Geometry: final body of the model. Coordinates: model frame, mm. A direction names the side the tool comes from. Coordinates: 2 decimals unless noted, no trailing zeros. Write each loop counter-clockwise with the first axis right and the second up, starting at its lowest first coordinate (ties: lowest second). Pieces come first, ordered by that corner, then holes. Notation, with made-up numbers: (-10, 21) -> (-3, 21) arc R12 cw to (-3, 43) -> close; hole circle Ø4 at (-23.5, 57). An arc over 180 degrees is marked (long way). One line per item, written item: value. Start each with the question number.
from build123d import *

# Parameters (mm, degrees)
SKETCH1_R           = 73.025
SKETCH1_R_2         = 42.926
BOSS_EXTRUDE1_DEPTH = 38.1
SKETCH2_R           = 69.088
CUT_EXTRUDE1_DEPTH  = 30.226
SKETCH4_R           = 5.588
BOSS_EXTRUDE2_DEPTH = 7.874
SKETCH4_3_R         = 5.588
CUT_EXTRUDE2_DEPTH  = 111.076842478
SKETCH4_4_R         = 5.588
CUT_EXTRUDE3_DEPTH  = 111.076842478


with BuildPart() as part:
    # Sketch1 → Boss-Extrude1 (new body)
    with BuildSketch(Plane(origin=(0, 0, 0), x_dir=(1, 0, 0), z_dir=(0, 1, 0))):
        with Locations(Location((0, 0, 0), (0, 0, 90))):
            Circle(SKETCH1_R)
        with Locations(Location((0, 0, 0), (0, 0, 90))):
            Circle(SKETCH1_R_2, mode=Mode.SUBTRACT)
    extrude(amount=BOSS_EXTRUDE1_DEPTH)

    # Sketch2 → Cut-Extrude1 (cut)
    with BuildSketch(Plane(origin=(0, 38.1, 0), x_dir=(1, 0, 0), z_dir=(0, 1, 0))):
        with Locations(Location((0, 0, 0), (0, 0, 270))):
            Circle(SKETCH2_R)
    extrude(amount=-CUT_EXTRUDE1_DEPTH, mode=Mode.SUBTRACT)

    # Sketch4 → Boss-Extrude2 (add)
    # profile 1 of 4: a face of its own
    with BuildSketch(Plane(origin=(0, 38.1, 0), x_dir=(1, 0, 0), z_dir=(0, 1, 0))):
        with BuildLine():
            Line((-58.01806662, 11.176), (-68.17806662, 11.176))
            ThreePointArc((-68.17806662, 11.176), (-69.088, 0), (-68.17806662, -11.176))
            Line((-68.17806662, -11.176), (-58.01806662, -11.176))
            ThreePointArc((-58.01806662, -11.176), (-46.84206662, 0), (-58.01806662, 11.176))
        make_face()
        with Locations(Location((-58.01806662, 0, 0), (0, 0, 270))):
            Circle(SKETCH4_R, mode=Mode.SUBTRACT)
    # profile 2 of 4: a face of its own
    with BuildSketch(Plane(origin=(0, 38.1, 0), x_dir=(1, 0, 0), z_dir=(0, 1, 0))):
        with BuildLine():
            ThreePointArc((11.177, 68.177902688), (0.001013346, 69.087999993), (-11.175, 68.178230536))
            Line((-11.175, 68.178230536), (-11.175, 58.01906662))
            ThreePointArc((-11.175, 58.01906662), (0.001, 46.84306662), (11.177, 58.01906662))
            Line((11.177, 58.01906662), (11.177, 68.177902688))
        make_face()
        with Locations(Location((0, 58.01806662, 0), (0, 0, 270))):
            Circle(SKETCH4_R, mode=Mode.SUBTRACT)
    # profile 3 of 4: a face of its own
    with BuildSketch(Plane(origin=(0, 38.1, 0), x_dir=(1, 0, 0), z_dir=(0, 1, 0))):
        with BuildLine():
            ThreePointArc((69.088, 0), (68.860140904, 5.606490764), (68.17806662, 11.176))
            Line((68.17806662, 11.176), (58.02006662, 11.176))
            ThreePointArc((58.02006662, 11.176), (46.84406662, 0), (58.02006662, -11.176))
            Line((58.02006662, -11.176), (68.17806662, -11.176))
            ThreePointArc((68.17806662, -11.176), (68.860140904, -5.606490764), (69.088, 0))
        make_face()
        with Locations(Location((58.01806662, 0, 0), (0, 0, 270))):
            Circle(SKETCH4_R, mode=Mode.SUBTRACT)
    # profile 4 of 4: a face of its own
    with BuildSketch(Plane(origin=(0, 38.1, 0), x_dir=(1, 0, 0), z_dir=(0, 1, 0))):
        with BuildLine():
            Line((-11.175, -58.01906662), (-11.175, -68.178230536))
            ThreePointArc((-11.175, -68.178230536), (0.001013346, -69.087999993), (11.177, -68.177902688))
            Line((11.177, -68.177902688), (11.177, -58.01906662))
            ThreePointArc((11.177, -58.01906662), (0.001, -46.84306662), (-11.175, -58.01906662))
        make_face()
        with Locations(Location((0, -58.01806662, 0), (0, 0, 270))):
            Circle(SKETCH4_R, mode=Mode.SUBTRACT)
    extrude(amount=-BOSS_EXTRUDE2_DEPTH)

    # Sketch4_3 → Cut-Extrude2 (cut, through all)
    with BuildSketch(Plane(origin=(0, 38.1, 0), x_dir=(1, 0, 0), z_dir=(0, 1, 0))):
        with Locations(Location((-41.024968338, 41.024968338, 0), (0, 0, 270))):
            Circle(SKETCH4_3_R)
        with Locations(Location((41.024968338, 41.024968338, 0), (0, 0, 270))):
            Circle(SKETCH4_3_R)
        with Locations(Location((41.024968338, -41.024968338, 0), (0, 0, 270))):
            Circle(SKETCH4_3_R)
        with Locations(Location((-41.024968338, -41.024968338, 0), (0, 0, 270))):
            Circle(SKETCH4_3_R)
    extrude(amount=-CUT_EXTRUDE2_DEPTH, mode=Mode.SUBTRACT)

    # Sketch4_4 → Cut-Extrude3 (cut, through all)
    with BuildSketch(Plane(origin=(0, 38.1, 0), x_dir=(1, 0, 0), z_dir=(0, 1, 0))):
        with Locations(Location((-58.01806662, 0, 0), (0, 0, 270))):
            Circle(SKETCH4_4_R)
        with Locations(Location((0, 58.01806662, 0), (0, 0, 270))):
            Circle(SKETCH4_4_R)
        with Locations(Location((58.01806662, 0, 0), (0, 0, 270))):
            Circle(SKETCH4_4_R)
        with Locations(Location((0, -58.01806662, 0), (0, 0, 270))):
            Circle(SKETCH4_4_R)
    extrude(amount=-CUT_EXTRUDE3_DEPTH, mode=Mode.SUBTRACT)


solid = part.part
Q1. Draft query along Y for faces 4 (the flat face through (-63, 34, -11.176)), 5 (the flat face through (65, 30.226, 0)), 6 (the flat face through (31, 0, -31)). Return one class per face: pulls with the +Y half, pulls with the -Y half, needs draft (parallel to the pull), parting line crosses it, or undercut.
Q2. Line query: L1, parallel to X at y = 34, z = 0 (3 decimals); L2, parallel to X at y = 3, z = 0 (3 decimals); L3, parallel to X at y = 8.5, z = -1. Output: solid intervals per line, ascending. Write a range as from..to.
Q3. Cut plane D-D on y = 33. Output: boundary loops of the cut face in (x, z) (3 decimals).
Q4. Access query for faces 1 (the cylindrical face through (-21.935, 18.783, -69.653)), 2 (the cylindrical face through (-0.245, 34.218, -46.846)), 3 (the flat face through (-3, 30.226, -63)). Directions: +Z, -Z, +X, -X, +Y, -Y. A direction counts if a zero-diameter tool reaches every point of the face in a straight line with its end or side. Return the directions, or none.
Q5. Cut plane A-A on x = 0. Count the separate pieces of the cut face and the enclosed holes in it, and give its area (3 significant figures).
Q6. Cut plane C-C on x = 49.5. Output: boundary loops of the cut face in (y, z).
Q7. First-contact query: P1, Ø8.5, axis at y = 34, z = 64.5, coming from the +X side; P2, Ø8, axis at y = 27, z = -14, coming from the -X side; P3, Ø8.5, axis at y = 35.5, z = -64, coming from the -X side. Flat tips, straight axial feed; report the tip coordinate or a pass-through.
Solution:
1. face 4: needs draft
1. face 5: undercut
1. face 6: pulls with the -Y half
2. L1: -73.025..-63.606, -52.43..-46.842, 46.844..52.43, 63.606..73.025
2. L2: -73.025..-63.606, -52.43..-42.926, 42.926..52.43, 63.606..73.025
2. L3: -73.02..-69.08, 69.08..73.02
3. outline: circle Ø146.05 at (0, 0); hole (-68.178, -11.176) arc R69.088 ccw to (-11.175, -68.178) -> (-11.175, -58.019) arc R11.176 cw to (11.177, -58.019) -> (11.177, -68.178) arc R69.088 ccw to (68.178, -11.176) -> (58.02, -11.176) arc R11.176 cw to (58.02, 11.176) -> (68.178, 11.176) arc R69.088 ccw to (11.177, 68.178) -> (11.177, 58.019) arc R11.176 cw to (-11.175, 58.019) -> (-11.175, 68.178) arc R69.088 ccw to (-68.178, 11.176) -> (-58.018, 11.176) arc R11.176 cw to (-58.018, -11.176) -> close; hole circle Ø11.176 at (-58.018, 0); hole circle Ø11.176 at (0, -58.018); hole circle Ø11.176 at (0, 58.018); hole circle Ø11.176 at (58.018, 0)
4. face 1: +Y, -Y
4. face 2: +Y
4. face 3: none
5. separate pieces: 6
5. enclosed holes: 0
5. area: 710 mm²
6. outline: (0, -53.69) -> (38.1, -53.69) -> (38.1, -48.2) -> (7.87, -48.2) -> (7.87, 48.2) -> (38.1, 48.2) -> (38.1, 53.69) -> (0, 53.69) -> close; (30.23, -7.23) -> (38.1, -7.23) -> (38.1, 7.23) -> (30.23, 7.23) -> close
7. P1: x = 41.26
7. P2: x = -72.34
7. P3: x = -41.98
